The listing builds one solid part. Answer for the finished solid, in the listing's coordinates (mm). Face numbers are marked on the shaded views. A direction names the side the tool comes from. Coordinates: 2 decimals unless noted, no trailing zeros. Order: outer loops, then holes, each group sorted by start corner. A loop starts at its lowest first (then second) coordinate and runs counter-clockwise, first axis right, second up. Notation, with made-up numbers: M 52,-7 L 63,-7 A22 cw 63,12 Z; hole C 66.5,-17.75 d4. An arc over 180 degrees is marked long. One line per item, written item: value. Start each with the question number.
Q1. The part is cut by section B-B on z = -2. Give the vertices of the cut face in (x, y), then the cut area to 3 significant figures.
Q2. The part is cut by section C-C on y = 240.5. Give the vertices of the cut face in (x, z).
Q3. The part is cut by section D-D on y = 0. Give the vertices of the cut face in (x, z).
Q4. Straight lines are drawn through the part: line 1 along Y through (x, z) = (6, 14); line 2 along Y through (x, z) = (35, -5.5); line 3 along X through (y, z) = (541, 10.5). For each, find the intervals that lie inside material, in ascending order. Write a range as [from, to].
Q5. The part is cut by section A-A on x = 13. Give the vertices of the cut face in (y, z).
Q6. For the marked faces 1, 2 and 3, determine the directions among +Z, -Z, +X, -X, +Y, -Y from which every point of the face is accessible in a straight line to the end or side of a thin tool.
Q7. Each of these flat-tipped pins is pushed along its axis until it touches: pin 1 Ø10 at (x, z) = (34, -4) entering from +Y; pin 2 Ø2 at (y, z) = (57, 9) entering from -X; pin 3 Ø6.5 at (y, z) = (582.5, 13.5) entering from -X. Where does it stop, or does it pass through?
```python
from build123d import *
from build123d.topology import SkipClean

# Parameters (mm, degrees)
BOSS_EXTRUDE1_DEPTH      = 11
BOSS_EXTRUDE1_DEPTH_BACK = 11
BOSS_EXTRUDE2_DEPTH      = 17
BOSS_EXTRUDE2_DEPTH_BACK = 17
SKETCH3_R                = 38


with BuildPart() as part:
    # Sketch1 → Boss-Extrude1 (new, two sides: drawn at the far end of the back side and taken through both)
    with BuildSketch(Plane.XY.offset(-BOSS_EXTRUDE1_DEPTH_BACK)):
        with BuildLine():
            Line((-28, 144), (-28, 25.690465157))
            ThreePointArc((-28, 25.690465157), (0, -38), (28, 25.690465157))
            Line((28, 25.690465157), (5, 65.527633731))
            Line((5, 65.527633731), (5, 144))
            Line((5, 144), (26.999618834, 226.103695235))
            Line((26.999618834, 226.103695235), (26.999618834, 431.103695235))
            Line((26.999618834, 431.103695235), (4.48236191, 515.139242122))
            Line((4.48236191, 515.139242122), (4.48236191, 553.98236191))
            Line((4.48236191, 553.98236191), (68, 617.5))
            Line((68, 617.5), (68, 645))
            Line((68, 645), (38, 645))
            Line((38, 645), (38, 705))
            ThreePointArc((38, 705), (-1.675998364, 742.96302187), (-37.852159447, 701.651265129))
            Line((-37.852159447, 701.651265129), (-28.51763809, 596.139242122))
            Line((-28.51763809, 596.139242122), (-28.51763809, 515.139242122))
            Line((-28.51763809, 515.139242122), (-6.000381166, 431.103695235))
            Line((-6.000381166, 431.103695235), (-6.000381166, 226.103695235))
            Line((-6.000381166, 226.103695235), (-28, 144))
        make_face()
    extrude(amount=BOSS_EXTRUDE1_DEPTH + BOSS_EXTRUDE1_DEPTH_BACK)

    # Sketch3 → Boss-Extrude2 (add, two sides: drawn at the far end of the back side and taken through both)
    with SkipClean():  # the faces are left unmerged after this step: merging them gives an invalid solid
        with BuildSketch(Plane.XY.offset(-BOSS_EXTRUDE2_DEPTH_BACK)):
            with Locations((0, 705)):
                Circle(SKETCH3_R)
            Circle(SKETCH3_R)
            Polygon((68, 617.5), (4.48236191, 553.98236191), (-12, 553.98236191), (-12, 645), (68, 645), align=None)
        extrude(amount=BOSS_EXTRUDE2_DEPTH + BOSS_EXTRUDE2_DEPTH_BACK)
    add(part.part.scale(1), mode=Mode.REPLACE)  # the faces are merged on a copy


solid = part.part
```
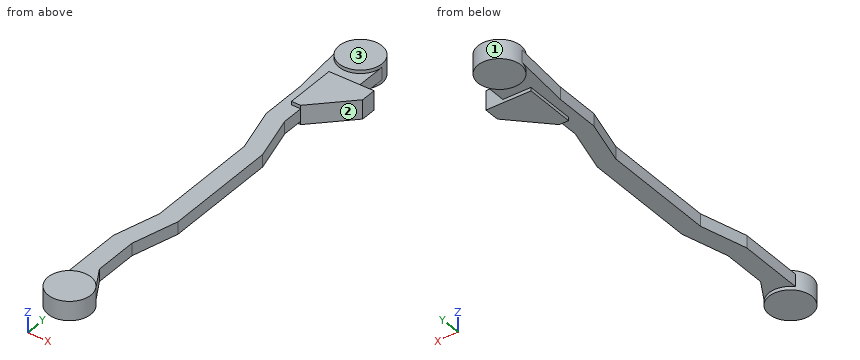
Output:
1. outline: M -37.85,701.65 L -28.52,596.14 L -28.52,515.14 L -6,431.1 L -6,226.1 L -28,144 L -28,25.69 A38 ccw long 28,25.69 L 5,65.53 L 5,144 L 27,226.1 L 27,431.1 L 4.48,515.14 L 4.48,553.98 L 68,617.5 L 68,645 L 38,645 L 38,705 A38 ccw long Z
1. area: 35,500 mm^2
2. outline: M -6,-11 L 27,-11 L 27,11 L -6,11 Z
3. outline: M -38,-17 L 38,-17 L 38,17 L -38,17 Z
4. line 1: y = [-37.52, 37.52], [555.5, 645], [667.48, 742.52]
4. line 2: y = [-14.8, 14.8], [584.5, 719.8]
4. line 3: x = [-28.52, 4.48]
5. outline: M -35.71,-17 L 35.71,-17 L 35.71,-11 L 51.67,-11 L 51.67,11 L 35.71,11 L 35.71,17 L -35.71,17 Z; M 173.86,-11 L 483.35,-11 L 483.35,11 L 173.86,11 Z; M 562.5,-17 L 645,-17 L 645,-11 L 669.29,-11 L 669.29,-17 L 740.71,-17 L 740.71,17 L 669.29,17 L 669.29,11 L 645,11 L 645,17 L 562.5,17 Z
6. face 1: none
6. face 2: +Z, -Z, +X
6. face 3: +Z, +X, -X, +Y, -Y
7. pin 1: stops at y = 729.56
7. pin 2: stops at x = -28
7. pin 3: stops at x = -28.52
